Autodesk Inventor part; units mm, degrees
ref_plane "YZ Plane" through (0, 0, 0) normal (1, 0, 0) x (0, 1, 0)
ref_plane "XZ Plane" through (0, 0, 0) normal (0, 1, 0) x (-1, 0, 0)
ref_plane "XY Plane" through (0, 0, 0) normal (0, 0, 1) x (1, 0, 0)
sketch "Esboço1" plane through (0, 0, 0) normal (0, 0, 1) x (1, 0, 0)
  circle A0 centre (0, 0) radius 1.2
  line L0 (0, 0) -> (0, 4.75) construction
  circle A1 centre (0, 4.75) radius 1.2
  dimension "d0" = 2.4
  dimension "d1" = 4.75
  dimension "d2" = 2.4
extrude "Extrusão1" add sketch "Esboço1" along normal blind 4
sketch "Esboço2" plane through (0, 4.75, 4) normal (0, 0, 1) x (1, 0, 0)
  circle A0 centre (0, -4.75) radius 1.2
  line L0 (0, -4.75) -> (0, -2.375) construction
  line L1 (0, -2.375) -> (-2, -2.375) construction
  line L2 (-2, -2.375) -> (-2, 2.625)
  line L3 (-2, -2.375) -> (-2, -7.375)
  line L4 (-2, 2.625) -> (154.4, 2.625)
  line L5 (-2, -7.375) -> (154.4, -7.375)
  line L6 (154.4, -7.375) -> (154.4, 2.625)
  dimension "d9" = 2.375
  dimension "d10" = 2
  dimension "d11" = 5
  dimension "d12" = 5
  dimension "d13" = 156.4
  dimension "d14" = 156.4
extrude "Extrusão2" add sketch "Esboço2" along normal blind 3 contours A0 | L2 L4 L6 L5 L3
sketch "Esboço3" plane through (0, 4.75, 4) normal (0, 0, -1) x (-1, 0, 0)
  circle A0 centre (0, 0) radius 1.2
  line L0 (0, 0) -> (0, 2.625) construction
  line L1 (-154.4, 2.625) -> (2, 2.625)
  line L2 (0, 2.625) -> (-4, 2.625) construction
  line L3 (-4, 2.625) -> (-4, 0.625)
  line L4 (-4, 0.625) -> (-154.4, 0.625)
  line L5 (-154.4, 0.625) -> (-154.4, 2.625)
  line L6 (-154.4, 2.625) -> (-4, 2.625)
  line L7 (2, 2.625) -> (2, -7.375)
  line L8 (2, -2.375) -> (-158, -2.375) construction
  line L9 (-4, -7.375) -> (-4, -5.375)
  line L10 (-4, -5.375) -> (-154.4, -5.375)
  line L11 (-154.4, -5.375) -> (-154.4, -7.375)
  line L12 (-154.4, -7.375) -> (-4, -7.375)
  point P0 (0, -4.75)
  dimension "d19" = 4
  dimension "d20" = 2
  dimension "d21" = 150.4
extrude "Extrusão3" add sketch "Esboço3" along normal blind 3 contours L1 L3 L4 L5 | L12 L11 L10 L9
sketch "Esboço4" plane through (-2, 7.375, 7) normal (0, 1, 0) x (1, 0, 0)
  line L0 (6, 3) -> (6, 6)
  line L1 (6, 4.5) -> (150.975, 4.5) construction
  line L2 (150.975, 4.5) -> (152.225, 4.5) construction
  line L3 (6, 3) -> (156.4, 3)
  line L4 (150.975, 4.5) -> (149.725, 4.5) construction
  line L5 (149.725, 5.5) -> (149.725, 6)
  line L6 (149.725, 6) -> (152.225, 6)
  line L7 (156.4, 6) -> (6, 6)
  line L8 (149.725, 6) -> (149.725, 5.5)
  line L9 (149.725, 5.5) -> (148.725, 5.5)
  line L10 (148.725, 5.5) -> (148.725, 4)
  line L11 (148.725, 4) -> (153.225, 4)
  line L12 (153.225, 4) -> (153.225, 5.5)
  line L13 (153.225, 5.5) -> (152.225, 5.5)
  line L14 (152.225, 5.5) -> (152.225, 6)
  point P0 (2, 7)
  point P1 (148.725, 4.5)
  point P2 (148.725, 3)
  point P3 (153.225, 3)
  dimension "d24" = 144.975
  dimension "d25" = 1.25
  dimension "d26" = 1.25
  dimension "d27" = 1
  dimension "d31" = 0.5
  dimension "d32" = 1.5
  dimension "d33" = 1
  dimension "d34" = 1.5
  dimension "d35" = 1
  dimension "d36" = 1
  dimension "d37" = 1
  dimension "d38" = 0.5
extrude "Extrusão4" cut sketch "Esboço4" against normal up to surface (10 mm away)
properties part number "Wiper-supportipt"
Geometry check sheet. Reference: the model listing, model coordinates, mm. A direction names the side the tool comes from. Round coordinates to 2 decimals unless told otherwise and drop trailing zeros. Loops run counter-clockwise (first coordinate to the right, second up) from the corner with the lowest first, then second, coordinate; pieces in that order, holes last.
Item 1: Access from +Z, -Z, +X, -X, +Y, -Y to the whole of each face (thin tool, end or side, straight path). Record for faces 5 (the cylindrical face through (0.65, 3.74, 1.97)), 6 (the flat face through (0, 5, 0)), 7 (the flat face through (78, -0.625, 3)).
Item 2: Thickness scan on line 1 (Y direction, x = 11, z = 2.25) (3 decimals); line 2 (Z direction, x = 43, y = -0.75); line 3 (Z direction, x = 5, y = 5). Record the ranges inside material, lowest first.
Item 3: Gauge pin test, flat ends, axial feed: pin 1 (0.6 mm diameter, centred on x = 149.5, y = 6.5, fed in from -Z); pin 2 (1.5 mm diameter, centred on y = -0.5, z = 1, fed in from -X); pin 3 (1.6 mm diameter, centred on x = 151.5, y = -1.5, fed in from -Z). Record the tip position at first contact, or that the pin passes through.
Item 4: Cross-section at A-A on x = 87. Record the boundary of the cut face in (y, z) (3 decimals), then the cut area to 3 significant figures.
Item 5: Mould release check, pull along Y, two halves, no side actions. Record for faces 1 (the flat face through (75, 2, 4)), 2 (the flat face through (75, 7.375, 4)), 3 (the flat face through (75, -2.625, 4)), 4 (the cylindrical face through (0.65, -1.01, 1.97)): pulls with the +Y half, pulls with the -Y half, needs draft (parallel to the pull), parting line crosses it, or undercut.
Answer sheet:
1. face 5: -Z
1. face 6: -Z, +X, -X, +Y, -Y
1. face 7: -Z, +X
2. line 1: y = -2.625 to -0.625, 5.375 to 7.375
2. line 2: z = 1 to 7
2. line 3: z = 4 to 7
3. pin 1: stops at z = 3
3. pin 2: stops at x = -1.2
3. pin 3: stops at z = 1
4. outline: (-2.625, 1) - (-0.625, 1) - (-0.625, 4) - (5.375, 4) - (5.375, 1) - (7.375, 1) - (7.375, 7) - (-2.625, 7) - close
4. area: 42.0 mm2
5. face 1: undercut
5. face 2: pulls with the +Y half
5. face 3: pulls with the -Y half
5. face 4: undercut
